For this review, take the finished solid that the model builds, in its own axes (mm). A direction names the side the tool comes from. Coordinates: 2 decimals unless noted, no trailing zeros. Order: outer loops, then holes, each group sorted by start corner. A loop starts at its lowest first (then second) coordinate and runs counter-clockwise, first axis right, second up.
from build123d import *

# Parameters (mm, degrees)
F0_W     = 6
F0_H     = 2
F1_DEPTH = 40
F0_R     = 1.25
F2_DEPTH = 2.5
F3_START = 37.5
F3_DEPTH = 2.5


with BuildPart() as f1:
    # F0 (on Front) → F1 (new body)
    with BuildSketch(Plane.XZ):
        with Locations((0, 9)):
            Rectangle(F0_W, F0_H)
    extrude(amount=F1_DEPTH)

    # F0 (on Front) → F2 (join)
    with BuildSketch(Plane.XZ):
        with BuildLine():
            Line((-3, 8), (-3, 0))
            ThreePointArc((-3, 0), (0, -3), (3, 0))
            Line((3, 0), (3, 8))
            Line((3, 8), (-3, 8))
        make_face()
        Circle(F0_R, mode=Mode.SUBTRACT)
    extrude(amount=F2_DEPTH)

    # F0 (on Front) → F3 (join)
    with BuildSketch(Plane.XZ.offset(F3_START)):
        with BuildLine():
            Line((-3, 8), (-3, 0))
            ThreePointArc((-3, 0), (0, -3), (3, 0))
            Line((3, 0), (3, 8))
            Line((3, 8), (-3, 8))
        make_face()
        Circle(F0_R, mode=Mode.SUBTRACT)
    extrude(amount=F3_DEPTH)


solid = f1.part
1. Take a section at A-A, the plane x = 0. Give the boundary of the cut face in (y, z).
Answer below:
outline: (-40, -3) - (-37.5, -3) - (-37.5, -1.25) - (-40, -1.25) - close; (-40, 1.25) - (-37.5, 1.25) - (-37.5, 8) - (-2.5, 8) - (-2.5, 1.25) - (0, 1.25) - (0, 10) - (-40, 10) - close; (-2.5, -3) - (0, -3) - (0, -1.25) - (-2.5, -1.25) - close
2. Take a section at D-D, the plane y = -25. Give the boundary of the cut face in (x, z).
Answer below:
outline: (-3, 8) - (3, 8) - (3, 10) - (-3, 10) - close
3. The part is to be moulded in two halves that separate along Y. For faces 1 (the face through (0, -20, 8)), 2 (the face through (3, -18.4, 8.3)), 3 (the face through (0, -40, 4)), say which applies: +Y half, -Y half, draft (parallel to the pull), parting line (faces both ways), or undercut.
Answer below:
face 1: undercut
face 2: draft
face 3: -Y half
4. Take a section at B-B, the plane z = 3.5. Give the boundary of the cut face in (x, y).
Answer below:
outline: (-3, -40) - (3, -40) - (3, -37.5) - (-3, -37.5) - close; (-3, -2.5) - (3, -2.5) - (3, 0) - (-3, 0) - close
5. Take a section at C-C, the plane x = -2.2. Give the boundary of the cut face in (y, z), plus the area to 3 significant figures.
Answer below:
outline: (-40, -2.04) - (-37.5, -2.04) - (-37.5, 8) - (-2.5, 8) - (-2.5, -2.04) - (0, -2.04) - (0, 10) - (-40, 10) - close
area: 130 mm2
6. Clearance check with a flat-ended pin moving along its axis: pin 1 Ø3 at (x, y) = (1, -26) entering from -Z. State where the tip first meets the part, or that it passes through.
Answer below:
pin 1: stops at z = 8
7. Machinability: for faces 4 (the face through (0, -37.5, 3)), 5 (the face through (0, -1, -3)), which of the approach directions +Z, -Z, +X, -X, +Y, -Y give a long, thin tool a straight path to every point of the face, cutting with its end or side? Answer none if there is none.
Answer below:
face 4: -Z, +X, -X
face 5: -Z, +Y, -Y
8. To check wall thickness, follow L1, parallel to Y at x = -0.6, z = 5; L2, parallel to Z at x = 0, y = -38.75; L3, parallel to Z at x = -1.9, y = -32. State the ranges of each line that lie inside material, in increasing order.
Answer below:
L1: y = -40 to -37.5, -2.5 to 0
L2: z = -3 to -1.25, 1.25 to 10
L3: z = 8 to 10
